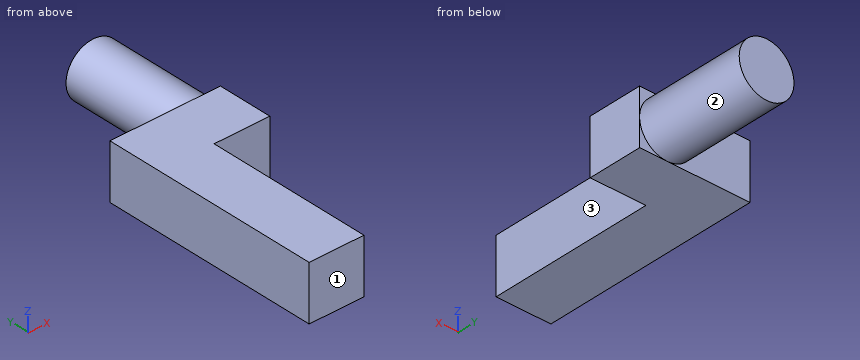
Autodesk Inventor part; units mm, degrees
ref_plane "YZ Plane" through (0, 0, 0) normal (1, 0, 0) x (0, 1, 0)
ref_plane "XZ Plane" through (0, 0, 0) normal (0, 1, 0) x (-1, 0, 0)
ref_plane "XY Plane" through (0, 0, 0) normal (0, 0, 1) x (1, 0, 0)
sketch "Sketch1" plane through (0, 0, 0) normal (0, 1, 0) x (-1, 0, 0)
  line L0 (-1.5748, 1.5748) -> (1.5748, 1.5748)
  line L1 (1.5748, 1.5748) -> (1.5748, -1.5748)
  line L2 (1.5748, -1.5748) -> (-1.5748, -1.5748)
  line L3 (-1.5748, -1.5748) -> (-1.5748, 1.5748)
  line L4 (-1.5748, 1.5748) -> (1.5748, -1.5748) construction
  line L5 (1.5748, 1.5748) -> (-1.5748, -1.5748) construction
  point P0 (0, 0)
  dimension "d0" = 3.1496
  dimension "d1" = 3.1496
extrude "Extrusion1" add sketch "Sketch1" along normal blind 6.35
sketch "Sketch2" plane through (-1.5748, 0, 1.5748) normal (0, 0, 1) x (1, 0, 0)
  line L0 (3.1496, 0) -> (0, 0)
  line L1 (3.1496, 0) -> (0, 0)
  line L2 (0, 0) -> (0, 12.7)
  line L3 (0, 12.7) -> (3.1496, 12.7)
  line L4 (3.1496, 12.7) -> (3.1496, 0)
  line L5 (0, 12.7) -> (6.35, 12.7)
  line L6 (6.35, 12.7) -> (6.35, 9.5504)
  line L7 (6.35, 9.5504) -> (0, 9.5504)
  line L8 (0, 9.5504) -> (0, 12.7)
  point P0 (1.5748, 0)
  point P1 (3.1496, 9.5504)
  dimension "d4" = 12.7
  dimension "d5" = 6.35
  dimension "d6" = 3.1496
extrude "Extrusion2" add sketch "Sketch2" against normal blind 3.1496
sketch "Sketch3" plane through (-1.5748, 12.7, 1.5748) normal (0, 1, 0) x (1, 0, 0)
  line L0 (0, 3.1496) -> (6.35, 3.1496)
  line L1 (6.35, 3.1496) -> (3.2004, 3.1496)
  line L2 (3.2004, 3.1496) -> (3.2004, 0)
  line L3 (3.2004, 0) -> (6.35, 0)
  line L4 (6.35, 0) -> (6.35, 3.1496)
  circle A0 centre (4.7752, 1.5748) radius 1.5748
  point P0 (1.5748, 1.5748)
  dimension "d9" = 3.1496
  dimension "d10" = 3.1496
extrude "Extrusion3" add sketch "Sketch3" along normal blind 6.35 contours A0
properties part number "Handle"
Check sheet for the modelled part. Datum: model origin and axes. Units: mm. Face numbers are marked on the shaded views. A direction names the side the tool comes from. Round coordinates to 2 decimals unless told otherwise and drop trailing zeros. Loops run counter-clockwise (first coordinate to the right, second up) from the corner with the lowest first, then second, coordinate; pieces in that order, holes last. Notation, with made-up numbers: (3.5, 18.25) - (60.5, 18.25) arc R22 ccw to (60.5, 32.25) - close; hole circle Ø8 at (59.25, 71). An arc over 180 degrees is marked (long way). Write item = value, one per line. Start each with the question number.
Q1. Section check D-D (z = -1). Record the boundary of the cut face in (x, y).
Q2. Section check A-A (z = 0.7). Record the boundary of the cut face in (x, y), plus the area to 3 significant figures.
Q3. Section check C-C (x = 2.75). Record the boundary of the cut face in (y, z), plus the area to 3 significant figures.
Q4. Access from +Z, -Z, +X, -X, +Y, -Y to the whole of each face (thin tool, end or side, straight path). Record for the marked faces 1, 2 and 3.
Q5. Section check B-B (y = 8.75). Record the boundary of the cut face in (x, z).
Q6. Thickness scan on L1, parallel to Y at x = 3.25, z = 1.1; L2, parallel to Y at x = 1, z = 1.15; L3, parallel to X at y = 3, z = 1.15. Record the ranges inside material, lowest first.
Derived:
q1.outline = (-1.57, 0) - (1.57, 0) - (1.57, 9.55) - (4.78, 9.55) - (4.78, 12.7) - (4.42, 12.7) - (4.42, 19.05) - (1.98, 19.05) - (1.98, 12.7) - (-1.57, 12.7) - close
q2.outline = (-1.57, 0) - (1.57, 0) - (1.57, 9.55) - (4.78, 9.55) - (4.78, 12.7) - (4.61, 12.7) - (4.61, 19.05) - (1.79, 19.05) - (1.79, 12.7) - (-1.57, 12.7) - close
q2.area = 68.0 mm^2
q3.outline = (9.55, -1.57) - (12.7, -1.57) - (12.7, -1.51) - (19.05, -1.51) - (19.05, 1.51) - (12.7, 1.51) - (12.7, 1.57) - (9.55, 1.57) - close
q3.area = 29.1 mm^2
q4.face_1 = +Z, -Z, +X, -X, -Y
q4.face_2 = +Y
q4.face_3 = +Z, -Z, +X, -Y
q5.outline = (-1.57, -1.57) - (1.57, -1.57) - (1.57, 1.57) - (-1.57, 1.57) - close
q6.L1 = 9.55 to 19.05
q6.L2 = 0 to 12.7
q6.L3 = -1.57 to 1.57
